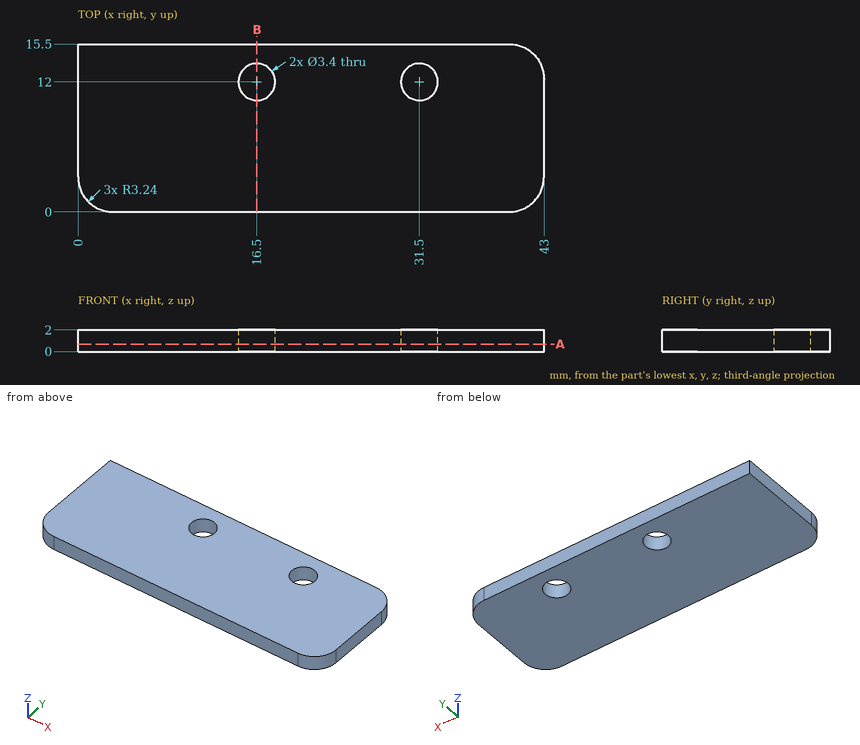
The drawing under review shows one solid part. Ordinate dimensions are in mm from its lowest x, y, z. Round coordinates to 2 decimals unless told otherwise and drop trailing zeros. Order: outer loops, then holes, each group sorted by start corner. A loop starts at its lowest first (then second) coordinate and runs counter-clockwise, first axis right, second up. Notation, with made-up numbers: (15.5, 3.25) -> (38.5, 3.25) arc R21 cw to (38.5, 13.25) -> close; hole circle Ø11 at (37.25, -4.75). An arc over 180 degrees is marked (long way). Use a Markdown table: item, result.
Item 1: For line 1 along Y through (x, z) = (16.5, 0.4); line 2 along X through (y, z) = (12.75, 0.4); line 3 along Y through (x, z) = (30.5, 1.2), list the stretches that pass through material, from the lowest coordinate up. Write a range as [from, to].
Resolved:
| item | result |
|---|---|
| line 1 | y = [0, 10.3], [13.7, 15.5] |
| line 2 | x = [0, 14.97], [18.03, 29.97], [33.03, 42.96] |
| line 3 | y = [0, 10.63], [13.37, 15.5] |
Item 2: For pin 1 (2 mm diameter, centred on x = 16.5, y = 12, fed in from +Z), flat-tipped, find the tip position at first contact; note if it passes through.
Resolved:
| item | result |
|---|---|
| pin 1 | passes through |
Item 3: Take a section at A-A (z = 0.7). State the section outline as (x, y) points, plus the area to 3 significant figures.
Resolved:
| item | result |
|---|---|
| outline | (0, 3.24) arc R3.24 ccw to (3.24, 0) -> (39.76, 0) arc R3.24 ccw to (43, 3.24) -> (43, 12.26) arc R3.24 ccw to (39.76, 15.5) -> (0, 15.5) -> close; hole circle Ø3.4 at (16.5, 12); hole circle Ø3.4 at (31.5, 12) |
| area | 642 mm² |
Item 4: Take a section at B-B (x = 16.5). State the section outline as (y, z) points, plus the area to 3 significant figures.
Resolved:
| item | result |
|---|---|
| outline | (0, 0) -> (10.3, 0) -> (10.3, 2) -> (0, 2) -> close; (13.7, 0) -> (15.5, 0) -> (15.5, 2) -> (13.7, 2) -> close |
| area | 24.2 mm² |
